Geometry: final body of the model. Coordinates: model frame, mm. A direction names the side the tool comes from. Round coordinates to 2 decimals unless told otherwise and drop trailing zeros. Order: outer loops, then holes, each group sorted by start corner. A loop starts at its lowest first (then second) coordinate and runs counter-clockwise, first axis right, second up. Notation, with made-up numbers: (64.25, -18) -> (87.25, -18) arc R17 cw to (87.25, -12) -> close; hole circle Ø11 at (53.5, 59). An arc over 180 degrees is marked (long way). Put each result on its own line as item: value.
```python
from build123d import *

# Parameters (mm, degrees)
F0_W        = 61.4208132029
F0_H        = 40.0461480021
F0_R        = 5.8356598506
F0_R_2      = 5.6623382773
F1_DEPTH    = 25.4
F2_T1_DEPTH = 86.8208132029


# Not quite as in the source:
# - a fillet or chamfer that OpenCascade refuses, or shapes differently, is made with other operations: its cross-section is extruded or revolved along the edge and cut away or added


with BuildPart() as f1:
    # F0 (on Top) → F1 (new body)
    with BuildSketch(Plane.XY):
        with Locations((9.6422955394, -0.2926178277)):
            Rectangle(F0_W, F0_H)
        with BuildLine():
            ThreePointArc((-15.5581902422, 6.5874267261), (-13.0892777006, 4.4019793182), (-9.8877530545, 3.6133415997))
            ThreePointArc((-9.8877530545, 3.6133415997), (-9.3918088824, 3.1173974276), (-9.8877530545, 2.6214532554))
            ThreePointArc((-9.8877530545, 2.6214532554), (-13.525571131, 3.5108261592), (-16.3427069667, 5.9783046702))
            ThreePointArc((-16.3427069667, 5.9783046702), (-16.2723997648, 6.6975216235), (-15.5581902422, 6.5874267261))
        make_face(mode=Mode.SUBTRACT)
        with BuildLine():
            ThreePointArc((-5.9691235315, 4.8356190614), (-3.7836761236, 7.304531603), (-2.9950384051, 10.5060562491))
            ThreePointArc((-2.9950384051, 10.5060562491), (-2.4990942329, 11.0020004213), (-2.0031500608, 10.5060562491))
            ThreePointArc((-2.0031500608, 10.5060562491), (-2.8925229646, 6.8682381727), (-5.3600014756, 4.051102337))
            ThreePointArc((-5.3600014756, 4.051102337), (-6.0792184289, 4.1214095389), (-5.9691235315, 4.8356190614))
        make_face(mode=Mode.SUBTRACT)
        with BuildLine():
            ThreePointArc((-13.8063825775, 16.1764934369), (-15.9918299854, 13.7075808953), (-16.7804677039, 10.5060562491))
            ThreePointArc((-16.7804677039, 10.5060562491), (-17.2764118761, 10.010112077), (-17.7723560482, 10.5060562491))
            ThreePointArc((-17.7723560482, 10.5060562491), (-16.8829831444, 14.1438743256), (-14.4155046334, 16.9610101613))
            ThreePointArc((-14.4155046334, 16.9610101613), (-13.6962876801, 16.8907029594), (-13.8063825775, 16.1764934369))
        make_face(mode=Mode.SUBTRACT)
        with Locations((-9.8877530545, 10.5060562491)):
            Circle(F0_R, mode=Mode.SUBTRACT)
        with BuildLine():
            ThreePointArc((-9.8877530545, 17.3987708986), (-10.3836972266, 17.8947150707), (-9.8877530545, 18.3906592429))
            ThreePointArc((-9.8877530545, 18.3906592429), (-6.249934978, 17.5012863391), (-3.4327991423, 15.0338078281))
            ThreePointArc((-3.4327991423, 15.0338078281), (-3.5031063442, 14.3145908748), (-4.2173158668, 14.4246857722))
            ThreePointArc((-4.2173158668, 14.4246857722), (-6.6862284084, 16.6101331801), (-9.8877530545, 17.3987708986))
        make_face(mode=Mode.SUBTRACT)
        with BuildLine():
            ThreePointArc((6.6644512117, 17.5767932087), (8.5373270865, 17.0581119265), (8.5140671581, 15.1148792356))
            ThreePointArc((8.5140671581, 15.1148792356), (4.0257871944, 13.7216332626), (1.5243776143, 9.7430981696))
            ThreePointArc((1.5243776143, 9.7430981696), (-0.0147844439, 10.1939229676), (0, 11.7976823822))
            ThreePointArc((0, 11.7976823822), (2.6892272592, 15.4287413311), (6.6644512117, 17.5767932087))
        make_face(mode=Mode.SUBTRACT)
        with Locations((9.6422955394, 6.0194581747)):
            Circle(F0_R_2, mode=Mode.SUBTRACT)
        Polygon((28.9662275463, 1.5064948219), (29.8360027373, 0), (28.9662275463, -1.5064948219), (27.2266771644, -1.5064948219), (26.3569019735, 0), (27.2266771644, 1.5064948219), align=None, mode=Mode.SUBTRACT)
        Polygon((33.9459068477, 1.8158181313), (31.6559560597, 1.8676351756), (30.5558555424, 3.8766992536), (31.7457058131, 5.8339462873), (34.0356566012, 5.782129243), (35.1357571185, 3.773065165), align=None, mode=Mode.SUBTRACT)
        Polygon((30.2401456875, 6.7547236703), (30.8922100812, 5.3890366107), (30.0355225909, 4.141488751), (28.5267707068, 4.259627951), (27.874706313, 5.6253150105), (28.7313938034, 6.8728628702), align=None, mode=Mode.SUBTRACT)
    extrude(amount=F1_DEPTH)

    # F2: fillet of radius 5.08 on 1 edges, made by hand

    # F2_s2 → F2_t1 (cut)
    with BuildSketch(Plane.YZ.offset(-33.768111062)):
        with BuildLine():
            ThreePointArc((19.7304561734, 20.32), (18.2425586218, 23.9121024484), (14.6504561734, 25.4))
            Line((14.6504561734, 25.4), (19.7304561734, 25.4))
            Line((19.7304561734, 25.4), (19.7304561734, 20.32))
        make_face()
    extrude(amount=F2_T1_DEPTH, mode=Mode.SUBTRACT)


solid = f1.part
```
1. Cut plane B-B on z = 7.75. State how many separate pieces and enclosed holes the cut face has, and give its area (3 significant figures).
Ans:
separate pieces: 1
enclosed holes: 10
area: 2,170 mm²
2. Draft query along Y for faces 1 (the face through (29.475, 6.815, 12.522)), 2 (the face through (-21.068, -1, 13)). Return one class per face: +Y half, -Y half, draft (parallel to the pull), parting line (faces both ways), or undercut.
Ans:
face 1: undercut
face 2: draft
3. Cut plane A-A on y = 12.5. Return loops of the section in (x, z), and give its area (3 significant figures).
Ans:
outline: (-21.07, 0) -> (-17.52, 0) -> (-17.52, 25.4) -> (-21.07, 25.4) -> close; (-16.49, 0) -> (-15.37, 0) -> (-15.37, 25.4) -> (-16.49, 25.4) -> close; (-4.4, 0) -> (0.34, 0) -> (0.34, 25.4) -> (-4.4, 25.4) -> close; (2.8, 0) -> (40.35, 0) -> (40.35, 25.4) -> (2.8, 25.4) -> close
area: 1,190 mm²
4. Contact query for flat-ended pins moving along their axis: P1, Ø9.5, axis at x = -9.89, y = 10.51, coming from the -Z side; P2, Ø13, axis at x = 9.64, y = 6.02, coming from the -Z side. Output: stop coordinate, or through.
Ans:
P1: through
P2: z = 0
5. Set-up query: faces 3 (the face through (40.353, -1, 13)), 4 (the face through (-3.805, 7.263, 12.522)). Return all of +Z, -Z, +X, -X, +Y, -Y with unobstructed straight access to the full face (end or side cutting, diameter ignored); none if empty.
Ans:
face 3: +Z, -Z, +X, +Y, -Y
face 4: +Z, -Z
6. Material intervals for probe 1 along X at (y, z) = (15.5, 5); probe 2 along Y at (x, z) = (33.5, 8.25); probe 3 along X at (y, z) = (0, 14.5), sorted ascending.
Ans:
probe 1: -21.07 to -15.99, -14.64 to -12.91, -6.87 to -5.14, -3.79 to 2.77, 8.74 to 40.35
probe 2: -20.32 to 1.83, 5.79 to 19.73
probe 3: -21.07 to 26.36, 29.84 to 40.35
